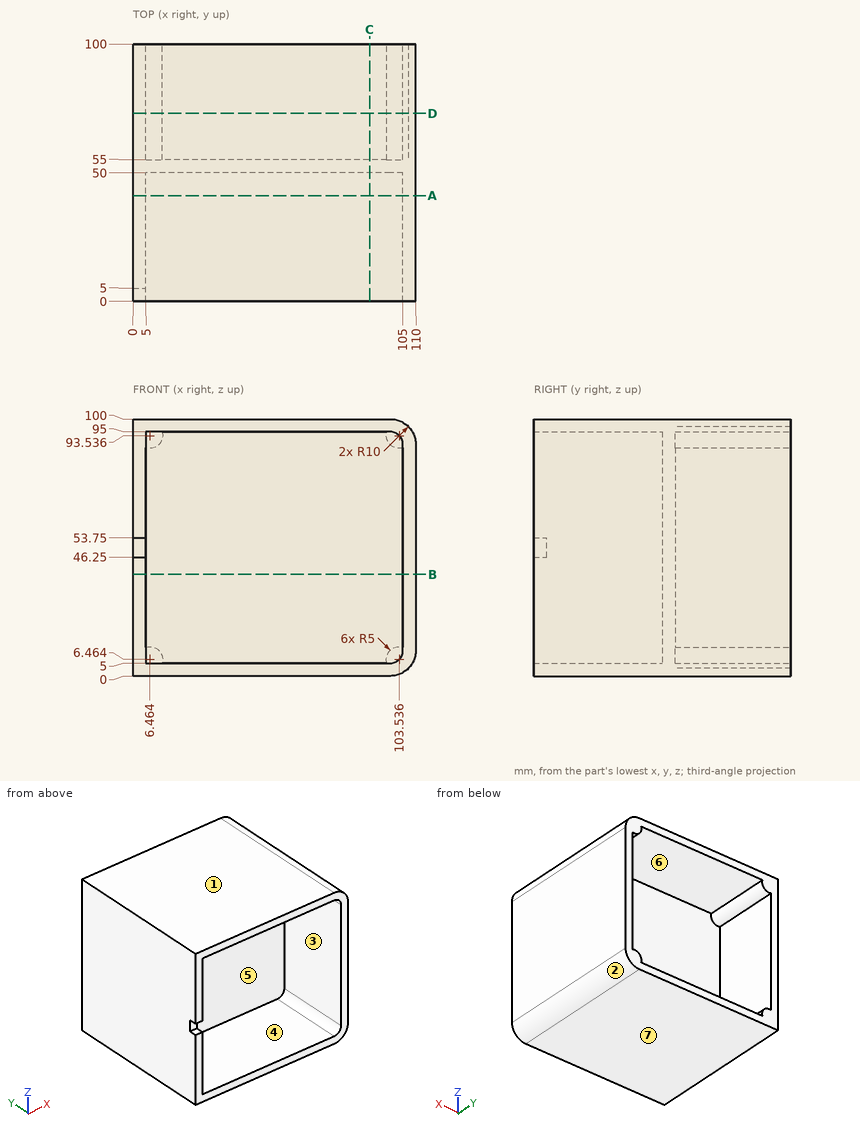
Geometry: see drawing. Coordinates: mm, zero at the bounding-box minimum. A direction names the side the tool comes from. Coordinates: 2 decimals unless noted, no trailing zeros. Loops run counter-clockwise (first coordinate to the right, second up) from the corner with the lowest first, then second, coordinate; pieces in that order, holes last. Notation, with made-up numbers: M 54.25,88 L 102.25,88 A10 ccw 102.25,101 Z; hole C 14.25,-32.5 d3. An arc over 180 degrees is marked long. Answer in a Markdown table with one row per item.
1. Draft query along X for the marked faces 1, 2, 3 and 4. Return one class per face: pulls with the +X half, pulls with the -X half, needs draft (parallel to the pull), parting line crosses it, or undercut.
Response:
| item | result |
|---|---|
| face 1 | needs draft |
| face 2 | pulls with the +X half |
| face 3 | undercut |
| face 4 | undercut |
2. Material intervals for line 1 (Z direction, x = 87, y = 60); line 2 (X direction, y = 12.5, z = 80.5); line 3 (Z direction, x = 8, y = 76), sorted ascending.
Response:
| item | result |
|---|---|
| line 1 | z = 0 to 5, 95 to 100 |
| line 2 | x = 0 to 5, 105 to 110 |
| line 3 | z = 0 to 11.22, 88.78 to 100 |
3. Section B-B, the plane z = 39.5. Output: boundary loops of the cut face in (x, y), then the cut area to 3 significant figures.
Response:
| item | result |
|---|---|
| outline | M 0,0 L 5,0 L 5,50 L 105,50 L 105,0 L 110,0 L 110,100 L 105,100 L 105,55 L 5,55 L 5,100 L 0,100 Z |
| area | 1,500 mm2 |
4. Reachability of the marked faces 5, 6 and 7 from +Z, -Z, +X, -X, +Y, -Y: full face, straight path, thin tool, end or side. Return the list, or none.
Response:
| item | result |
|---|---|
| face 5 | -Y |
| face 6 | +Y |
| face 7 | -Z, +X, -X, +Y, -Y |
5. Section D-D, the plane y = 73. Output: boundary loops of the cut face in (x, z) (1 decimal).
Response:
| item | result |
|---|---|
| outline | M 0,0 L 100,0 A10 ccw 110,10 L 110,90 A10 ccw 100,100 L 0,100 Z; hole M 5,11.2 A5 cw 11.2,5 L 98.8,5 A5 cw 105,11.2 L 105,88.8 A5 cw 98.8,95 L 11.2,95 A5 cw 5,88.8 Z |
6. Section A-A, the plane y = 41. Output: boundary loops of the cut face in (x, z).
Response:
| item | result |
|---|---|
| outline | M 0,0 L 100,0 A10 ccw 110,10 L 110,90 A10 ccw 100,100 L 0,100 Z; hole M 5,5 L 100,5 A5 ccw 105,10 L 105,90 A5 ccw 100,95 L 5,95 Z |
7. Section C-C, the plane x = 92. Output: boundary loops of the cut face in (y, z).
Response:
| item | result |
|---|---|
| outline | M 0,0 L 100,0 L 100,5 L 55,5 L 55,95 L 100,95 L 100,100 L 0,100 L 0,95 L 50,95 L 50,5 L 0,5 Z |
8. First-contact query: pin 1 (22.5 mm diameter, centred on y = 72, z = 48.5, fed in from -X); pin 2 (1.5 mm diameter, centred on x = 67.5, z = 53.5, fed in from +Y); pin 3 (5.5 mm diameter, centred on x = 1.5, z = 50, fed in from -Y); pin 4 (1.5 mm diameter, centred on x = 12, z = 84, fed in from -Y). Flat tips, straight axial feed; report the tip coordinate or a pass-through.
Response:
| item | result |
|---|---|
| pin 1 | stops at x = 0 |
| pin 2 | stops at y = 55 |
| pin 3 | stops at y = 5 |
| pin 4 | stops at y = 50 |
